Can you work these out from the model? Positions are in its coordinate system, mm. Face numbers are marked on the shaded views. A direction names the side the tool comes from. Give positions to 0.01 mm unless a question says otherwise; leave off trailing zeros. Order: outer loops, then holes, each group sorted by start corner. A loop starts at its lowest first (then second) coordinate and runs counter-clockwise, first axis right, second up. Notation, with made-up numbers: (28.5, -10) - (63.5, -10) arc R16 ccw to (63.5, 19) - close; hole circle Ø3 at (-16.5, 61.5). An arc over 180 degrees is marked (long way). Answer as CSV lines item,"result".
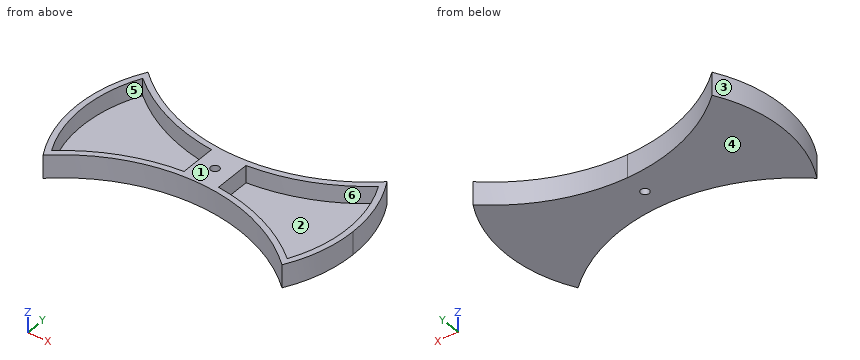
```python
from build123d import *

# Parameters (mm, degrees)
F1_DEPTH = 25.4
F3_DEPTH = 19.05
F4_R     = 4.6355
F5_DEPTH = 25.4


with BuildPart() as f1:
    # F0 (on Top) → F1 (new body)
    with BuildSketch(Plane.XY):
        with BuildLine():
            ThreePointArc((131.9822715367, -76.2), (147.2070959265, -39.4440224736), (152.4, 0))
            ThreePointArc((152.4, 0), (147.2070959265, 39.4440224736), (131.9822715368, 76.2))
            ThreePointArc((131.9822715367, 76.2), (70.7106074079, 38.5384530031), (0, 25.4))
            ThreePointArc((0, 25.4), (-70.7106074079, 38.5384530031), (-131.9822715367, 76.2))
            ThreePointArc((-131.9822715368, 76.2), (-152.4, 0), (-131.9822715367, -76.2))
            ThreePointArc((-131.9822715367, -76.2), (0, -25.4), (131.9822715367, -76.2))
        make_face()
    extrude(amount=F1_DEPTH)

    # F2 (on face) → F3 (cut)
    with BuildSketch(Plane.XY.offset(25.4)):
        with BuildLine():
            ThreePointArc((-19.05, 19.9449395097), (-78.1175048106, 34.6656311359), (-130.1742098035, 66.2214285714))
            ThreePointArc((-130.1742098035, 66.2214285714), (-146.05, 0), (-130.1742098035, -66.2214285714))
            ThreePointArc((-130.1742098035, -66.2214285714), (-78.1175048106, -34.6656311359), (-19.05, -19.9449395097))
            Line((-19.05, -19.9449395097), (-19.05, 0))
            Line((-19.05, 0), (-19.05, 19.9449395097))
        make_face()
        with BuildLine():
            ThreePointArc((19.05, -19.9449395097), (78.1175048106, -34.6656311359), (130.1742098035, -66.2214285714))
            ThreePointArc((130.1742098035, -66.2214285714), (146.05, 0), (130.1742098035, 66.2214285714))
            ThreePointArc((130.1742098035, 66.2214285714), (78.1175048106, 34.6656311359), (19.05, 19.9449395097))
            Line((19.05, 19.9449395097), (19.05, 0))
            Line((19.05, 0), (19.05, -19.9449395097))
        make_face()
    extrude(amount=-F3_DEPTH, mode=Mode.SUBTRACT)

    # F4 (on face) → F5 (cut, through all)
    with BuildSketch(Plane.XY.offset(25.4)):
        Circle(F4_R)
    extrude(amount=-F5_DEPTH, mode=Mode.SUBTRACT)


solid = f1.part
```
1) I want a section at C-C on x = 111.5. Write out the boundary of the cut face in (y, z).
Answer block:
outline,"(-60.02, 0) - (60.02, 0) - (60.02, 25.4) - (52.37, 25.4) - (52.37, 6.35) - (-52.37, 6.35) - (-52.37, 25.4) - (-60.02, 25.4) - close"
2) I want a section at A-A on z = 10. Write out the boundary of the cut face in (x, y), plus the area to 3 significant figures.
Answer block:
outline,"(-131.98, -76.2) arc R196.85 cw to (131.98, -76.2) arc R152.4 ccw to (131.98, 76.2) arc R196.85 cw to (-131.98, 76.2) arc R152.4 ccw to start; hole (-130.17, -66.22) arc R203.2 cw to (-19.05, -19.94) - (-19.05, 19.94) arc R203.2 cw to (-130.17, 66.22) arc R146.05 ccw to start; hole circle Ø9.27 at (0, 0); hole (19.05, -19.94) arc R203.2 cw to (130.17, -66.22) arc R146.05 ccw to (130.17, 66.22) arc R203.2 cw to (19.05, 19.94) - close"
area,"6,920 mm2"
3) I want a section at D-D on x = -96.5. Write out the boundary of the cut face in (y, z), plus the area to 3 significant figures.
Answer block:
outline,"(-50.68, 0) - (50.68, 0) - (50.68, 25.4) - (43.43, 25.4) - (43.43, 6.35) - (-43.43, 6.35) - (-43.43, 25.4) - (-50.68, 25.4) - close"
area,"920 mm2"
4) If we mould it in two halves opening along Y, with no side actions, what happens to the marked faces 3, 4, 5 and 6? For each: +Y half, -Y half, draft (parallel to the pull), parting line (faces both ways), or undercut.
Answer block:
face 3,"parting line"
face 4,"draft"
face 5,"undercut"
face 6,"undercut"
5) I need wall thicknesses on line 1 along X through (y, z) = (65, 8.75); line 2 along Z through (x, y) = (102, 32); line 3 along Y through (x, z) = (-69, 16.5). Which ranges of each line are inside material? Lowest first, please. Write a range as [from, to].
Answer block:
line 1,"[-137.84, -130.79], [-128.7, -118.42], [118.42, 128.7], [130.79, 137.84]"
line 2,"[0, 6.35]"
line 3,"[-37.89, -31.12], [31.12, 37.89]"
6) Which directions (+Z, -Z, +X, -X, +Y, -Y) give clear straight access to the entire face, cutting with the end or side of a thin tool? Please do the marked faces 1 and 2.
Answer block:
face 1,"+Z, +X, -X, +Y, -Y"
face 2,"+Z"
7) I want a section at B-B on y = 36.5. Write out the boundary of the cut face in (x, z).
Answer block:
outline,"(-147.96, 0) - (-65.17, 0) - (-65.17, 25.4) - (-82.38, 25.4) - (-82.38, 6.35) - (-141.42, 6.35) - (-141.42, 25.4) - (-147.96, 25.4) - close; (65.17, 0) - (147.96, 0) - (147.96, 25.4) - (141.42, 25.4) - (141.42, 6.35) - (82.38, 6.35) - (82.38, 25.4) - (65.17, 25.4) - close"
8) I'm going to push flat-ended pins straight in: P1, Ø6, axis at x = -95, z = 10, coming from the +Y side; P2, Ø3, axis at x = 120.5, z = 15.5, coming from the -Y side; P3, Ø8, axis at y = -59, z = 21.5, coming from the -X side. Where does each tip first touch, or does it pass through?
Answer block:
P1,"y = 51.53"
P2,"y = -67.76"
P3,"x = -142.13"
